Here's how the part is built. I have some questions about the finished solid (model axes, mm). Face numbers are marked on the shaded views. A direction names the side the tool comes from. Coordinates: 2 decimals unless noted, no trailing zeros. Loops run counter-clockwise (first coordinate to the right, second up) from the corner with the lowest first, then second, coordinate; pieces in that order, holes last. Notation, with made-up numbers: (-35, 35.25) - (-15, 35.25) arc R20 ccw to (-15, 63.25) - close; hole circle Ø7 at (55.5, -10). An arc over 180 degrees is marked (long way). Use a Markdown table: item, result.
```python
from build123d import *

# Parameters (mm, degrees)
F0_W     = 84
F0_H     = 40
F0_W_2   = 30.2
F0_H_2   = 14.2
F1_DEPTH = 25
F2_W     = 30.2
F2_H     = 14.2
F3_DEPTH = 23
F5_DEPTH = 5
F6_R     = 1
F7_DEPTH = 5
F8_W     = 11
F8_H     = 9
F8_H_2   = 5
F9_DEPTH = 1.5


with BuildPart() as f1:
    # F0 (on Top) → F1 (new body)
    with BuildSketch(Plane.XY):
        Rectangle(F0_W, F0_H)
        Rectangle(F0_W_2, F0_H_2, mode=Mode.SUBTRACT)
    extrude(amount=F1_DEPTH)

    # F2 (on face) → F3 (cut)
    with BuildSketch(Plane.XY.offset(25)):
        with BuildLine():
            Line((-37.2087121525, -18.5), (37.2087121525, -18.5))
            ThreePointArc((37.2087121525, -18.5), (37.732233047, -15.732233047), (40.5, -15.2087121525))
            Line((40.5, -15.2087121525), (40.5, 15.2087121525))
            ThreePointArc((40.5, 15.2087121525), (37.732233047, 15.732233047), (37.2087121525, 18.5))
            Line((37.2087121525, 18.5), (-37.2087121525, 18.5))
            ThreePointArc((-37.2087121525, 18.5), (-37.0527342177, 18.0107741092), (-37, 17.5))
            ThreePointArc((-37, 17.5), (-38.1306936062, 15.4083499337), (-40.5, 15.2087121525))
            Line((-40.5, 15.2087121525), (-40.5, -15.2087121525))
            ThreePointArc((-40.5, -15.2087121525), (-38.1306936062, -15.4083499337), (-37, -17.5))
            ThreePointArc((-37, -17.5), (-37.0527342177, -18.0107741092), (-37.2087121525, -18.5))
        make_face()
        Rectangle(F2_W, F2_H, mode=Mode.SUBTRACT)
    extrude(amount=-F3_DEPTH, mode=Mode.SUBTRACT)

    # F4 (on face) → F5 (join)
    with BuildSketch(Plane.XY.offset(2)):
        with BuildLine():
            Line((-15.1, 7.1), (-13.6, 7.1))
            ThreePointArc((-13.6, 7.1), (-16.1606601718, 8.1606601718), (-15.1, 5.6))
            Line((-15.1, 5.6), (-15.1, 7.1))
        make_face()
        with BuildLine():
            Line((-15.1, -7.1), (-15.1, -5.6))
            ThreePointArc((-15.1, -5.6), (-16.1606601718, -8.1606601718), (-13.6, -7.1))
            Line((-13.6, -7.1), (-15.1, -7.1))
        make_face()
        with BuildLine():
            ThreePointArc((13.6, -7.1), (16.1606601718, -8.1606601718), (15.1, -5.6))
            Line((15.1, -5.6), (15.1, -7.1))
            Line((15.1, -7.1), (13.6, -7.1))
        make_face()
        with BuildLine():
            ThreePointArc((15.1, 5.6), (16.1606601718, 8.1606601718), (13.6, 7.1))
            Line((13.6, 7.1), (15.1, 7.1))
            Line((15.1, 7.1), (15.1, 5.6))
        make_face()
    extrude(amount=F5_DEPTH)

    # F6 (on face) → F7 (cut)
    with BuildSketch(Plane.XY.offset(25)):
        with Locations((-39.5, 17.5)):
            Circle(F6_R)
        with Locations((39.5, 17.5)):
            Circle(F6_R)
        with Locations((39.5, -17.5)):
            Circle(F6_R)
        with Locations((-39.5, -17.5)):
            Circle(F6_R)
    extrude(amount=-F7_DEPTH, mode=Mode.SUBTRACT)

    # F8 (on face) → F9 (cut, through all)
    with BuildSketch(Plane.XZ.offset(20)):
        with Locations((-6.5, 15.5)):
            Rectangle(F8_W, F8_H)
        with Locations((-6.5, 22.5)):
            Rectangle(F8_W, F8_H_2)
    extrude(amount=-F9_DEPTH, mode=Mode.SUBTRACT)


solid = f1.part
```
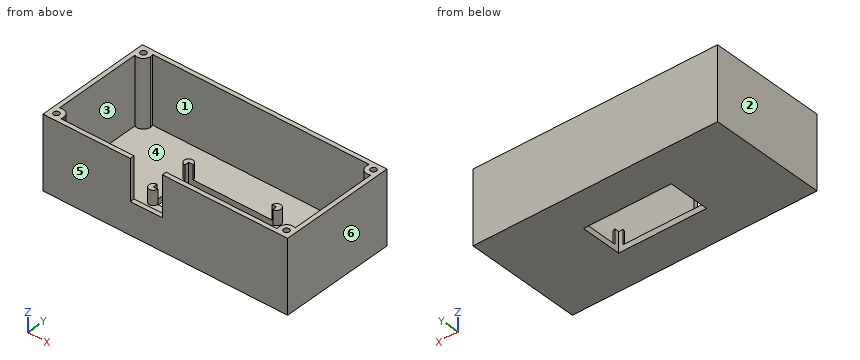
Q1. Which directions (+Z, -Z, +X, -X, +Y, -Y) give clear straight access to the entire face, cutting with the end or side of a thin tool? Please do the marked faces 1 and 2.
Check values:
| item | result |
|---|---|
| face 1 | +Z |
| face 2 | +Z, -Z, -X, +Y, -Y |
Q2. Will these pins go through, and if not, where does the flat tip stop? P1, Ø10, axis at x = -15, y = 3.5, coming from the +Z side; P2, Ø1.6, axis at x = -39.5, y = -17.5, coming from the +Z side; P3, Ø10, axis at x = -33, y = 8.5, coming from the +Z side.
Check values:
| item | result |
|---|---|
| P1 | z = 7 |
| P2 | z = 20 |
| P3 | z = 2 |
Q3. I want a section at C-C, the plane x = -39.5. Write out the boundary of the cut face in (y, z), then the cut area to 3 significant figures.
Check values:
| item | result |
|---|---|
| outline | (-20, 0) - (20, 0) - (20, 25) - (18.5, 25) - (18.5, 20) - (16.5, 20) - (16.5, 25) - (15, 25) - (15, 2) - (-15, 2) - (-15, 25) - (-16.5, 25) - (-16.5, 20) - (-18.5, 20) - (-18.5, 25) - (-20, 25) - close |
| area | 290 mm^2 |
Q4. Please list where these lines run through material, in increasing order: L1, parallel to Y at x = -39.5, z = 23.8; L2, parallel to Y at x = -9, z = 2.5; L3, parallel to Z at x = 29, y = -16.5. Write a range as from..to.
Check values:
| item | result |
|---|---|
| L1 | -20..-18.5, -16.5..-15, 15..16.5, 18.5..20 |
| L2 | -20..-18.5, 18.5..20 |
| L3 | 0..2 |
Q5. I want a section at D-D, the plane y = -10.5. Write out the boundary of the cut face in (x, z).
Check values:
| item | result |
|---|---|
| outline | (-42, 0) - (42, 0) - (42, 25) - (40.5, 25) - (40.5, 2) - (-40.5, 2) - (-40.5, 25) - (-42, 25) - close |
Q6. I want a section at B-B, the plane y = 2. Write out the boundary of the cut face in (x, z), then the cut area to 3 significant figures.
Check values:
| item | result |
|---|---|
| outline | (-42, 0) - (-15.1, 0) - (-15.1, 2) - (-40.5, 2) - (-40.5, 25) - (-42, 25) - close; (15.1, 0) - (42, 0) - (42, 25) - (40.5, 25) - (40.5, 2) - (15.1, 2) - close |
| area | 177 mm^2 |
Q7. I want a section at A-A, the plane x = -4.5. Write out the boundary of the cut face in (y, z).
Check values:
| item | result |
|---|---|
| outline | (-20, 0) - (-7.1, 0) - (-7.1, 2) - (-18.5, 2) - (-18.5, 11) - (-20, 11) - close; (7.1, 0) - (20, 0) - (20, 25) - (18.5, 25) - (18.5, 2) - (7.1, 2) - close |
Q8. If we mould it in two halves opening along X, with no side actions, what happens to the marked faces 3, 4, 5 and 6? For each: pulls with the +X half, pulls with the -X half, needs draft (parallel to the pull), parting line crosses it, or undercut.
Check values:
| item | result |
|---|---|
| face 3 | undercut |
| face 4 | undercut |
| face 5 | needs draft |
| face 6 | pulls with the +X half |
